```python
from build123d import *

# Parameters (mm, degrees)
SKETCH1_R           = 2.3
SKETCH1_R_2         = 2.5
BOSS_EXTRUDE1_DEPTH = 3


with BuildPart() as part:
    # Sketch1 → Boss-Extrude1 (new body)
    with BuildSketch(Plane.XY):
        with BuildLine():
            Line((-11.5, 21), (2, 21))
            Line((2, 21), (2, -2))
            Line((2, -2), (-1.360059051, -2))
            ThreePointArc((-1.360059051, -2), (-1.348623714, -11.019912453), (-4.688647717, -19.398646909))
            ThreePointArc((-4.688647717, -19.398646909), (-5.126699638, -21.05045095), (-4.522206104, -22.648866929))
            Line((-4.522206104, -22.648866929), (-3.277176831, -24.214083243))
            ThreePointArc((-3.277176831, -24.214083243), (-4.144083243, -31.822823169), (-11.752823169, -30.955916757))
            Line((-11.752823169, -30.955916757), (-12.538462624, -29.968232598))
            ThreePointArc((-12.538462624, -29.968232598), (-18.164899658, -32.689735637), (-24.264648783, -34.05224549))
            ThreePointArc((-24.264648783, -34.05224549), (-27.093039229, -34.2), (-29.921429675, -34.05224549))
            ThreePointArc((-29.921429675, -34.05224549), (-51.958319855, -17.944091524), (-48.851858813, 9.175035542))
            ThreePointArc((-48.851858813, 9.175035542), (-48.800272502, 9.340767339), (-48.864085593, 9.502186251))
            Line((-48.864085593, 9.502186251), (-49.933529172, 10.732440358))
            ThreePointArc((-49.933529172, 10.732440358), (-49.399336437, 18.371752377), (-41.760024419, 17.837559642))
            Line((-41.760024419, 17.837559642), (-40.69058084, 16.607305535))
            ThreePointArc((-40.69058084, 16.607305535), (-40.095055579, 16.303481207), (-39.455414432, 16.49795167))
            ThreePointArc((-39.455414432, 16.49795167), (-33.463302383, 19.841462143), (-26.7, 21))
            Line((-26.7, 21), (-22.5, 21))
            Line((-22.5, 21), (-22.5, 26.353946086))
            ThreePointArc((-22.5, 26.353946086), (-17, 31.853946086), (-11.5, 26.353946086))
            Line((-11.5, 26.353946086), (-11.5, 21))
        make_face()
        with Locations((-45.846776795, 14.285)):
            Circle(SKETCH1_R, mode=Mode.SUBTRACT)
        with Locations((-7.515, -27.585)):
            Circle(SKETCH1_R, mode=Mode.SUBTRACT)
        with Locations((-17, 26.353946086)):
            Circle(SKETCH1_R_2, mode=Mode.SUBTRACT)
    extrude(amount=BOSS_EXTRUDE1_DEPTH)


solid = part.part
```
Could you check a few things on this model? Use its own coordinates, in mm. A direction names the side the tool comes from. Round coordinates to 2 decimals unless told otherwise and drop trailing zeros. Write each loop counter-clockwise with the first axis right and the second up, starting at its lowest first coordinate (ties: lowest second). Pieces come first, ordered by that corner, then holes. Notation, with made-up numbers: M 44.25,-13.75 L 103.25,-13.75 A25 cw 103.25,24.25 Z; hole C -32,-12 d1. An arc over 180 degrees is marked long. Write each question's results on one line, items separated by ' | '. Start each with the question number.
1. Imagine slicing it at C-C on y = 6.5. List the corners of the cut face in (x, z) for me.
2. Thinking about a two-plate mould opening in X: for faces 4 (the face through (-26, -8, 0)), 5 (the face through (-22.5, 24, 1)), 6 (the face through (2, 10, 1)), 7 (the face through (-49.49, 18.29, 1.48)), which applies, +X half, -X half, draft (parallel to the pull), parting line (faces both ways), or undercut?
3. I'm going to push flat-ended pins straight in: pin 1 Ø0.9 at (x, z) = (0.5, 1.5) entering from -Y; pin 2 Ø1 at (y, z) = (-17, 0.5) entering from -X; pin 3 Ø1.5 at (y, z) = (25, 1.5) entering from -X. Where does each tip first touch, or does it pass through?
4. Imagine slicing it at B-B on z = 2.2. Count the separate pieces of the cut face and the enclosed holes in it, and give its area (3 significant figures).
5. On a 3-axis mill with a long thin cutter (end or side, diameter ignored), from which of +Z, -Z, +X, -X, +Y, -Y can I reach the whole of each face in a straight line? I mean faces 1 (the face through (-11.5, 24, 1)), 2 (the face through (-33.55, 19.81, 1.48)), 3 (the face through (-3.91, -23.42, 1.48)). Say none if no direction works.
6. Imagine slicing it at A-A on x = -17. List the corners of the cut face in (y, z) for me, and give its area (3 significant figures).
7. I need wall thicknesses on L1, parallel to X at y = 17.5, z = 2.6; L2, parallel to X at y = 21.5, z = 1.9; L3, parallel to Y at x = -17, z = 0.9. Which ranges of each line are inside material? Lowest first, please. Write a range as from..to.
8. Imagine slicing it at D-D on y = -9. List the corners of the cut face in (x, z) for me.
Result sheet:
1) outline: M -50.61,0 L 2,0 L 2,3 L -50.61,3 Z
2) face 4: draft | face 5: -X half | face 6: +X half | face 7: undercut
3) pin 1: stops at y = -2 | pin 2: stops at x = -52.54 | pin 3: stops at x = -22.5
4) separate pieces: 1 | enclosed holes: 3 | area: 2,700 mm^2
5) face 1: +Z, -Z, +X, +Y | face 2: +Z, -Z, +Y | face 3: +Z, -Z, +X
6) outline: M -32.25,0 L 23.85,0 L 23.85,3 L -32.25,3 Z; M 28.85,0 L 31.85,0 L 31.85,3 L 28.85,3 Z | area: 177 mm^2
7) L1: x = -50.2..-41.47, -38.1..2 | L2: x = -22.5..-11.5 | L3: y = -32.25..23.85, 28.85..31.85
8) outline: M -54.17,0 L -1.05,0 L -1.05,3 L -54.17,3 Z
